```python
from build123d import *

# Parameters (mm, degrees)
F0_W     = 140
F0_H     = 60
F1_DEPTH = 60
F3_R     = 10
F5_DEPTH = 69
F4_R     = 10
F6_DEPTH = 9.8


with BuildPart() as f1:
    # F0 (on Top) → F1 (new body)
    with BuildSketch(Plane.XY):
        Rectangle(F0_W, F0_H)
    extrude(amount=F1_DEPTH)

    # F3 (on Top) → F5 (join)
    with BuildSketch(Plane.XY):
        with Locations((-50, 0)):
            Circle(F3_R)
    extrude(amount=F5_DEPTH)

    # F4 (on face) → F6 (cut)
    with BuildSketch(Plane.XY.offset(60)):
        with Locations((50, 0)):
            Circle(F4_R)
    extrude(amount=-F6_DEPTH, mode=Mode.SUBTRACT)


solid = f1.part
```
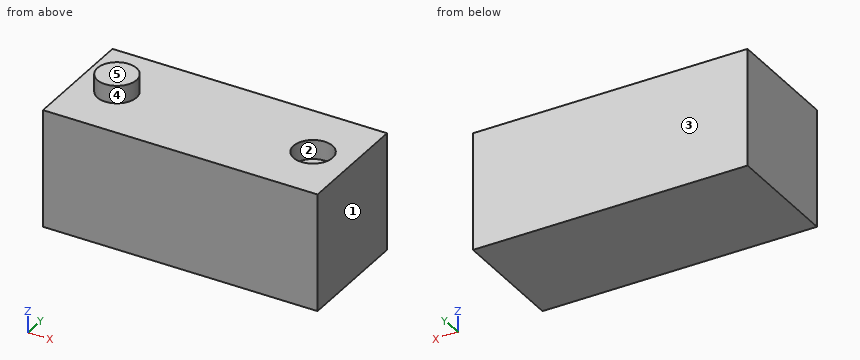
Part model, mm, in its own coordinate system. Face numbers are marked on the shaded views. A direction names the side the tool comes from. Coordinates: 2 decimals unless noted, no trailing zeros. Loops run counter-clockwise (first coordinate to the right, second up) from the corner with the lowest first, then second, coordinate; pieces in that order, holes last. Notation, with made-up numbers: (78.25, 63.5) - (97.25, 63.5) arc R18 ccw to (97.25, 78.5) - close; hole circle Ø8 at (-40, 42.5). An arc over 180 degrees is marked (long way). Write item = value, one per line. Start each with the question number.
Item 1: 3-axis set-ups, long thin cutter, end or side, ignore diameter. For the marked faces 4 and 5: which of +Z, -Z, +X, -X, +Y, -Y reach the whole face in a straight line?
Item 2: Cut at C-C, the plane z = 53. Give the cut face in (x, y), and give its area (3 significant figures).
Item 3: Cut at D-D, the plane x = 50. Give the cut face in (y, z).
Item 4: Flat gauge pins, fed straight in: pin 1 Ø6 at (x, y) = (47, 1) entering from +Z; pin 2 Ø18 at (x, y) = (12, 4) entering from +Z. Where does each tip first touch, or does it go through?
Item 5: Cut at B-B, the plane x = -50. Give the cut face in (y, z).
Item 6: Mould opens along X. For the marked faces 1, 2 and 3 say: released by +X, released by -X, zero draft, split by the parting line, or undercut.
Item 7: Cut at A-A, the plane y = 0. Give the cut face in (x, z).
Item 8: Wall check: L1, parallel to Y at x = 50, z = 52.75; L2, parallel to Z at x = 7.5, y = 26.5; L3, parallel to Y at x = -49.5, z = 61. Give the ranges that are in metal, low to high. Write a range as from..to.
The answers:
q1.face_4 = +Z
q1.face_5 = +Z, +X, -X, +Y, -Y
q2.outline = (-70, -30) - (70, -30) - (70, 30) - (-70, 30) - close; hole circle Ø20 at (50, 0)
q2.area = 8,090 mm2
q3.outline = (-30, 0) - (30, 0) - (30, 60) - (10, 60) - (10, 50.2) - (-10, 50.2) - (-10, 60) - (-30, 60) - close
q4.pin_1 = 50.2
q4.pin_2 = 60
q5.outline = (-30, 0) - (30, 0) - (30, 60) - (10, 60) - (10, 69) - (-10, 69) - (-10, 60) - (-30, 60) - close
q6.face_1 = released by +X
q6.face_2 = undercut
q6.face_3 = zero draft
q7.outline = (-70, 0) - (70, 0) - (70, 60) - (60, 60) - (60, 50.2) - (40, 50.2) - (40, 60) - (-40, 60) - (-40, 69) - (-60, 69) - (-60, 60) - (-70, 60) - close
q8.L1 = -30..-10, 10..30
q8.L2 = 0..60
q8.L3 = -9.99..9.99
